Autodesk Inventor part; units mm, degrees
ref_plane "YZ Plane" through (0, 0, 0) normal (1, 0, 0) x (0, 1, 0)
ref_plane "XZ Plane" through (0, 0, 0) normal (0, 1, 0) x (-1, 0, 0)
ref_plane "XY Plane" through (0, 0, 0) normal (0, 0, 1) x (1, 0, 0)
sketch "Szkic1" plane through (0, 0, 0) normal (0, 1, 0) x (-1, 0, 0)
  line L0 (-2, 0) -> (-98, 0)
  line L1 (-100, 2) -> (-100, 16)
  line L2 (-98, 18) -> (-2, 18)
  line L3 (0, 16) -> (0, 2)
  circle A0 centre (-9, 9) radius 2.5
  circle A1 centre (-30, 9) radius 1.5
  circle A2 centre (-91, 9) radius 2.5
  circle A3 centre (-70, 9) radius 1.5
  arc A4 (-2, 0) -> (0, 2) centre (-2, 2) ccw
  arc A5 (0, 16) -> (-2, 18) centre (-2, 16) ccw
  arc A6 (-100, 2) -> (-98, 0) centre (-98, 2) ccw
  arc A7 (-98, 18) -> (-100, 16) centre (-98, 16) ccw
  point P0 (0, 0)
  point P1 (-100, 18)
  point P2 (-100, 0)
  point P3 (0, 18)
  dimension "d0" = 100
  dimension "d1" = 18
  dimension "d2" = 5
  dimension "d3" = 9
  dimension "d4" = 9
  dimension "d5" = 3
  dimension "d6" = 9
  dimension "d7" = 30
  dimension "d8" = 2
extrude "Wyciągnięcie proste1" add sketch "Szkic1" along normal blind 1.6
equation "\"d4\" = 0.5 * d1"
equation "\"d6\" = d4"
properties part number "ramie1a"
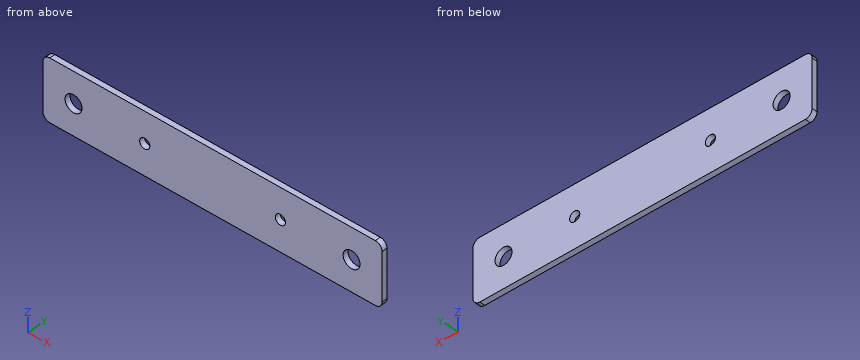
For this review, take the finished solid that the model builds, in its own axes (mm). Round coordinates to 2 decimals unless told otherwise and drop trailing zeros. Write each loop counter-clockwise with the first axis right and the second up, starting at its lowest first coordinate (ties: lowest second). Pieces come first, ordered by that corner, then holes.
1) Take a section at B-B on x = 91. Give the boundary of the cut face in (y, z), then the cut area to 3 significant figures.
Answer below:
outline: (0, 0) - (1.6, 0) - (1.6, 6.5) - (0, 6.5) - close; (0, 11.5) - (1.6, 11.5) - (1.6, 18) - (0, 18) - close
area: 20.8 mm2
2) Insertion check: pin 1 Ø2.5 at (x, z) = (70, 9) entering from +Y; pin 2 Ø5 at (x, z) = (30, 9) entering from +Y. Each pin has a flat end and moves straight along its axis. Give the tip position at first contact, or say it passes through.
Answer below:
pin 1: passes through
pin 2: stops at y = 1.6
3) Take a section at D-D on x = 70. Give the boundary of the cut face in (y, z).
Answer below:
outline: (0, 0) - (1.6, 0) - (1.6, 7.5) - (0, 7.5) - close; (0, 10.5) - (1.6, 10.5) - (1.6, 18) - (0, 18) - close
4) Take a section at A-A on z = 9. Give the boundary of the cut face in (x, y), then the cut area to 3 significant figures.
Answer below:
outline: (0, 0) - (6.5, 0) - (6.5, 1.6) - (0, 1.6) - close; (11.5, 0) - (28.5, 0) - (28.5, 1.6) - (11.5, 1.6) - close; (31.5, 0) - (68.5, 0) - (68.5, 1.6) - (31.5, 1.6) - close; (71.5, 0) - (88.5, 0) - (88.5, 1.6) - (71.5, 1.6) - close; (93.5, 0) - (100, 0) - (100, 1.6) - (93.5, 1.6) - close
area: 134 mm2
5) Take a section at C-C on y = 1.05. Give the boundary of the cut face in (x, z), then the cut area to 3 significant figures.
Answer below:
outline: (0, 2) arc R2 ccw to (2, 0) - (98, 0) arc R2 ccw to (100, 2) - (100, 16) arc R2 ccw to (98, 18) - (2, 18) arc R2 ccw to (0, 16) - close; hole circle Ø5 at (9, 9); hole circle Ø3 at (30, 9); hole circle Ø3 at (70, 9); hole circle Ø5 at (91, 9)
area: 1,740 mm2
6) For line 1 along X through (y, z) = (1.4, 8); line 2 along Z through (x, y) = (30, 1.35); line 3 along X through (y, z) = (0.1, 6.75), list the stretches that pass through material, from the lowest coordinate up.
Answer below:
line 1: x = 0 to 6.71, 11.29 to 28.88, 31.12 to 68.88, 71.12 to 88.71, 93.29 to 100
line 2: z = 0 to 7.5, 10.5 to 18
line 3: x = 0 to 7.91, 10.09 to 89.91, 92.09 to 100
